Could you check a few things on this model? Use its own coordinates, in mm. Face numbers are marked on the shaded views. A direction names the side the tool comes from. Round coordinates to 2 decimals unless told otherwise and drop trailing zeros. Write each loop counter-clockwise with the first axis right and the second up, starting at its lowest first coordinate (ties: lowest second). Pieces come first, ordered by that corner, then holes. Notation, with made-up numbers: M -37,29.5 L 8,29.5 A9 ccw 8,44.5 Z; hole C 27.25,-17.75 d9. An arc over 180 degrees is marked long. One line per question, with ' | ' between items. Start each with the question number.
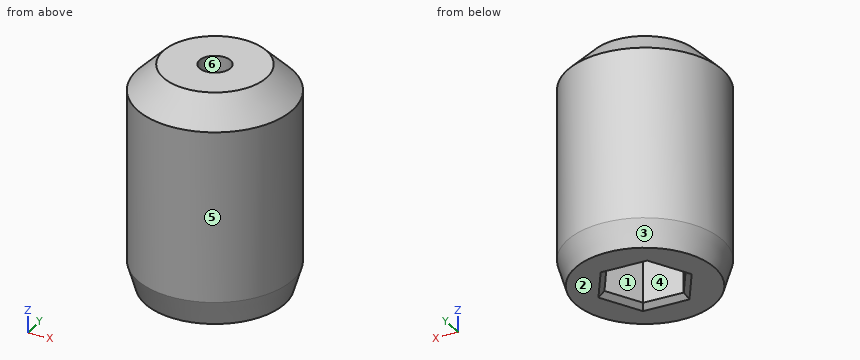
```python
from build123d import *

# Parameters (mm, degrees)
F0_R     = 15
F1_DEPTH = 18
F2_R     = 15
F2_R_2   = 3
F3_DEPTH = 25
F4_SIZE  = 5
F5_SIZE  = 1
F6_DEPTH = 1
F7_SIZE2 = 1.5
F7_SIZE  = 5


with BuildPart() as f1:
    # F0 (on Top) → F1 (new body)
    with BuildSketch(Plane.XY):
        Circle(F0_R)
        Polygon((-7.7942286341, 0), (-3.897114317, 6.75), (3.897114317, 6.75), (7.7942286341, 0), (3.897114317, -6.75), (-3.897114317, -6.75), align=None, mode=Mode.SUBTRACT)
    extrude(amount=F1_DEPTH)

    # F2 (on face) → F3 (join)
    with BuildSketch(Plane.XY.offset(18)):
        Circle(F2_R)
        Polygon((-3.897114317, -6.75), (-7.7942286341, 0), (-3.897114317, 6.75), (3.897114317, 6.75), (7.7942286341, 0), (3.897114317, -6.75), align=None, mode=Mode.SUBTRACT)
        Polygon((-3.897114317, 6.75), (-7.7942286341, 0), (-3.897114317, -6.75), (3.897114317, -6.75), (7.7942286341, 0), (3.897114317, 6.75), align=None)
        Circle(F2_R_2, mode=Mode.SUBTRACT)
    extrude(amount=F3_DEPTH)

    # F4
    f4_edges = [f1.edges().sort_by_distance(p)[0] for p in [
        (-15, 0, 43),
    ]]
    chamfer(f4_edges, length=F4_SIZE)

    # F5
    f5_edges = [f1.edges().sort_by_distance(p)[0] for p in [
        (0, -6.75, 0),
        (5.845671, -3.375, 0),
        (5.845671, 3.375, 0),
        (0, 6.75, 0),
        (-5.845671, 3.375, 0),
        (-5.845671, -3.375, 0),
    ]]
    chamfer(f5_edges, length=F5_SIZE)

    # F2 (on face) → F6 (join)
    with BuildSketch(Plane.XY.offset(18)):
        Circle(F2_R_2)
    extrude(amount=F6_DEPTH)

    # F7
    f7_edges = [f1.edges().sort_by_distance(p)[0] for p in [
        (-15, 0, 0),
    ]]
    f7_side = f1.faces().sort_by_distance((-15, 0, 19))[0]
    chamfer(f7_edges, length=F7_SIZE, length2=F7_SIZE2, reference=f7_side)


solid = f1.part
```
1. Which directions (+Z, -Z, +X, -X, +Y, -Y) give clear straight access to the entire face, cutting with the end or side of a thin tool? Please do the marked faces 4, 5 and 6.
2. I'm going to push flat-ended pins straight in: P1, Ø4, axis at y = -5.5, z = 18, coming from the +X side; P2, Ø8, axis at x = -7, z = 25, coming from the +Y side; P3, Ø12, axis at y = 8.5, z = 28.5, coming from the +X side. Where does each tip first touch, or does it pass through?
3. Suppose I cut it at B-B (x = 0). Write out the boundary of the cut face in (y, z), and give its area (4 significant figures).
4. Suppose I cut it at A-A (z = 12.5). Write out the boundary of the cut face in (x, y), and give its area (3 significant figures).
5. I need wall thicknesses on line 1 along Y through (x, z) = (0, 37); line 2 along Y through (x, z) = (0, 13.5); line 3 along X through (y, z) = (2, 33). Which ranges of each line are inside material? Lowest first, please. Write a range as from..to.
6. If we mould it in two halves opening along X, with no side actions, what happens to the marked faces 1, 2 and 3? For each: released by +X, released by -X, zero draft, split by the parting line, or undercut.
7. Suppose I cut it at C-C (z = 29). Write out the boundary of the cut face in (x, y), and give its area (3 significant figures).
Computed:
1) face 4: -Z | face 5: +Z, -Z | face 6: +Z
2) P1: stops at x = 14.59 | P2: stops at y = 14.7 | P3: stops at x = 14.79
3) outline: M -15,5 L -13.5,0 L -7.75,0 L -6.75,1 L -6.75,18 L 6.75,18 L 6.75,1 L 7.75,0 L 13.5,0 L 15,5 L 15,38 L 10,43 L 3,43 L 3,19 L -3,19 L -3,43 L -10,43 L -15,38 Z | area: 869.5 mm²
4) outline: C 0,0 d30; hole M -7.79,0 L -3.9,-6.75 L 3.9,-6.75 L 7.79,0 L 3.9,6.75 L -3.9,6.75 Z | area: 549 mm²
5) line 1: y = -15..-3, 3..15 | line 2: y = -15..-6.75, 6.75..15 | line 3: x = -14.87..-2.24, 2.24..14.87
6) face 1: undercut | face 2: zero draft | face 3: split by the parting line
7) outline: C 0,0 d30; hole C 0,0 d6 | area: 679 mm²
